```python
from build123d import *

# Parameters (mm, degrees)
SKETCH1_W               = 19
SKETCH1_H               = 19
BOSS_EXTRUDE1_DEPTH     = 7
FILLET1_R               = 9.5
SKETCH2_W               = 6
SKETCH2_H               = 19
BOSS_EXTRUDE2_DEPTH     = 15
FILLET2_R               = 7
SKETCH3_W               = 3
SKETCH3_H               = 5.02
CUT_EXTRUDE1_DEPTH      = 31.581857367
CUT_EXTRUDE2_DEPTH      = 27.367593747
CUT_EXTRUDE2_DEPTH_BACK = 27.367593747
SKETCH4_R               = 1.5
SKETCH5_R               = 2
CUT_EXTRUDE3_DEPTH      = 21.137030566


with BuildPart() as part:
    # Sketch1 → Boss-Extrude1 (new body)
    with BuildSketch(Plane(origin=(0, 0, 0), x_dir=(1, 0, 0), z_dir=(0, 1, 0))):
        Rectangle(SKETCH1_W, SKETCH1_H)
    extrude(amount=BOSS_EXTRUDE1_DEPTH)

    # Fillet1
    fillet1_edges = [part.edges().sort_by_distance(p)[0] for p in [
        (-9.5, 3.5, -9.5),
        (-9.5, 3.5, 9.5),
    ]]
    fillet(fillet1_edges, radius=FILLET1_R - 0.0001)  # a hair under: the kernel refuses the full size

    # Sketch2 → Boss-Extrude2 (add)
    with BuildSketch(Plane(origin=(0, 7, 0), x_dir=(1, 0, 0), z_dir=(0, 1, 0))):
        with Locations((6.5, 0)):
            Rectangle(SKETCH2_W, SKETCH2_H)
    extrude(amount=BOSS_EXTRUDE2_DEPTH)

    # Fillet2
    fillet2_edges = [part.edges().sort_by_distance(p)[0] for p in [
        (6.5, 22, -9.5),
        (6.5, 22, 9.5),
    ]]
    fillet(fillet2_edges, radius=FILLET2_R)

    # Sketch3 → Cut-Extrude1 (cut, through all)
    with BuildSketch(Plane(origin=(9.5, 0, 0), x_dir=(0, 0, -1), z_dir=(1, 0, 0))):
        with Locations((0, 11.26)):
            Rectangle(SKETCH3_W, SKETCH3_H)
    extrude(amount=-CUT_EXTRUDE1_DEPTH, mode=Mode.SUBTRACT)

    # Sketch4 → Cut-Extrude2 (cut, two sides: drawn at the far end of the back side and taken through both)
    with BuildSketch(Plane.XY.offset(-1.5).offset(-CUT_EXTRUDE2_DEPTH_BACK)):
        with Locations((7, 11.27)):
            Circle(SKETCH4_R)
    extrude(amount=CUT_EXTRUDE2_DEPTH + CUT_EXTRUDE2_DEPTH_BACK, mode=Mode.SUBTRACT)

    # Sketch5 → Cut-Extrude3 (cut, through all)
    with BuildSketch(Plane(origin=(0, 7, 0), x_dir=(1, 0, 0), z_dir=(0, 1, 0))):
        with Locations(Location((-2, 0, 0), (0, 0, 270))):
            Circle(SKETCH5_R)
    extrude(amount=-CUT_EXTRUDE3_DEPTH, mode=Mode.SUBTRACT)


solid = part.part
```
The model under review builds one solid part; all positions refer to its coordinate system, in mm. A direction names the side the tool comes from. Give positions to 0.01 mm unless a question says otherwise; leave off trailing zeros. Write each loop counter-clockwise with the first axis right and the second up, starting at its lowest first coordinate (ties: lowest second). Pieces come first, ordered by that corner, then holes. Notation, with made-up numbers: M 79,49.25 L 137,49.25 A37 ccw 137,88.25 Z; hole C -40,21 d4. An arc over 180 degrees is marked long. Answer in a Markdown table with one row per item.
Item 1: Draft analysis for pull direction X (two halves, no side actions). For faces 1 (the face through (-3.2, 3.5, -1.6)), 2 (the face through (6, 22, 0)), 3 (the face through (-6.791, 3.549, 6.643)), state which applies: +X half, -X half, draft (parallel to the pull), parting line (faces both ways), or undercut.
Check sheet entries:
| item | result |
|---|---|
| face 1 | undercut |
| face 2 | draft |
| face 3 | -X half |
Item 2: Add section A-A on y = 9.25. Give the boundary of the cut face in (x, z).
Check sheet entries:
| item | result |
|---|---|
| outline | M 3.5,-9.5 L 9.5,-9.5 L 9.5,-1.5 L 3.5,-1.5 Z; M 3.5,1.5 L 9.5,1.5 L 9.5,9.5 L 3.5,9.5 Z |
Item 3: Tool access review of faces 4 (the face through (5, 11, -1.5)), 5 (the face through (5.5, 11.3, -5.6)), 6 (the face through (-3, 7, 2)): name each direction out of +Z, -Z, +X, -X, +Y, -Y from which nothing blocks a thin tool from reaching the whole face with its end or side.
Check sheet entries:
| item | result |
|---|---|
| face 4 | +X, -X |
| face 5 | +Z, -Z |
| face 6 | +Z, -Z, -X, +Y |
Item 4: For line 1 along X through (y, z) = (5, 0); line 2 along X through (y, z) = (11.27, 7.75); line 3 along X through (y, z) = (15, 8.25), list the stretches that pass through material, from the lowest coordinate up.
Check sheet entries:
| item | result |
|---|---|
| line 1 | -9.5 to -4, 0 to 9.5 |
| line 2 | 3.5 to 5.5, 8.5 to 9.5 |
| line 3 | 3.5 to 9.5 |
Item 5: Add section D-D on z = -1. Give the boundary of the cut face in (x, y).
Check sheet entries:
| item | result |
|---|---|
| outline | M -9.45,0 L -3.73,0 L -3.73,7 L -9.45,7 Z; M -0.27,0 L 9.5,0 L 9.5,8.75 L 3.5,8.75 L 3.5,7 L -0.27,7 Z; M 3.5,13.77 L 9.5,13.77 L 9.5,22 L 3.5,22 Z |
Item 6: Add section B-B on x = -2.5. Give the boundary of the cut face in (y, z).
Check sheet entries:
| item | result |
|---|---|
| outline | M 0,-9.17 L 7,-9.17 L 7,-1.94 L 0,-1.94 Z; M 0,1.94 L 7,1.94 L 7,9.17 L 0,9.17 Z |
Item 7: For P1, Ø1, axis at x = -4.5, y = 5.5, coming from the +Z side; P2, Ø3, axis at x = 0.5, y = 16.5, coming from the +Z side; P3, Ø4.5, axis at y = 12, z = -4.5, coming from the -X side; P4, Ø1.5, axis at y = 7, z = 5.5, coming from the -X side, all flat-tipped, find the tip position at first contact; note any pin that passes through.
Check sheet entries:
| item | result |
|---|---|
| P1 | z = 8.62 |
| P2 | through |
| P3 | x = 3.5 |
| P4 | x = -8.23 |
